Model file for the job. Use its own axes, mm. A direction names the side the tool comes from. Round coordinates to 2 decimals unless told otherwise and drop trailing zeros. Order: outer loops, then holes, each group sorted by start corner. A loop starts at its lowest first (then second) coordinate and runs counter-clockwise, first axis right, second up. Notation, with made-up numbers: M -35,-38.75 L -3,-38.75 A32 ccw -3,-3.75 Z; hole C 62.25,85.5 d3. An arc over 180 degrees is marked long. Return JSON: item names as keys, results as strings. Group by question number.
Item 1: Slice it at C-C on z = 19.05. Write the cut outline in (x, y) (3 decimals).
Item 2: Which spindle directions (+Z, -Z, +X, -X, +Y, -Y) get a long thin tool onto all of the face, cutting with end or side? Do faces 4 (the face through (-3.746, 3.422, -0.165)), 5 (the face through (-0.37, -1.29, 2.85)), 6 (the face through (0, 15.875, 19)). Say none if no direction does.
Item 3: Probe line 1 along Z through (x, y) = (0, 2.15) (3 decimals); line 2 along Z through (x, y) = (0, 3.1) (3 decimals); line 3 along Z through (x, y) = (0, 3.25) (3 decimals). List the from-to ranges inside material, lowest first.
Item 4: Slice it at D-D on y = 13.75. Write the cut outline in (x, z) (3 decimals), then the cut area to 3 significant figures.
Item 5: Pull direction Z, two halves, no side cores. Call faces 1 (the face through (0, 3.175, 7)), 2 (the face through (-4.42, 1.57, 9.59)), 3 (the face through (-1, 3.675, -3)): pulls with the +Z half, pulls with the -Z half, needs draft (parallel to the pull), parting line crosses it, or undercut.
Item 6: Pin check, flat tips, straight feed: pin 1 Ø6 at (x, z) = (-0.5, 1) entering from +Y (3 decimals); pin 2 Ø4.5 at (x, z) = (1, -0.5) entering from -Y; pin 3 Ø5 at (y, z) = (12, 18) entering from +X (3 decimals); pin 4 Ø3 at (y, z) = (5, 3) entering from -X. Stop position of each tip, or through.
Item 7: Slice it at B-B on y = 1. Write the cut outline in (x, z) (3 decimals), then the cut area to 3 significant figures.
Item 8: Slice it at A-A on x = 0. Write the cut outline in (y, z) (3 decimals).
from build123d import *

# Parameters (mm, degrees)
SKETCH1_R           = 1.5
BOSS_EXTRUDE1_DEPTH = 3.175
SKETCH2_R           = 3.75
SKETCH2_R_2         = 2.75
BOSS_EXTRUDE2_DEPTH = 0.5
SKETCH3_R           = 2.75
SKETCH3_R_2         = 1.5
CUT_EXTRUDE1_DEPTH  = 0.8
SKETCH4_R           = 4.5
SKETCH4_R_2         = 2.5
BOSS_EXTRUDE3_DEPTH = 3.048
SKETCH5_R           = 2.875
CUT_EXTRUDE3_DEPTH  = 3.048
SKETCH6_R           = 3.175
BOSS_EXTRUDE4_DEPTH = 12.7
FILLET1_R           = 0.508


with BuildPart() as part:
    # Sketch1 → Boss-Extrude1 (new body)
    with BuildSketch(Plane(origin=(0, 0, 0), x_dir=(1, 0, 0), z_dir=(0, 1, 0))):
        with BuildLine():
            Line((-5.656854249, 0), (-3.148946712, -19.45590591))
            ThreePointArc((-3.148946712, -19.45590591), (0, -22.225), (3.148946712, -19.45590591))
            Line((3.148946712, -19.45590591), (5.656854249, 0))
            ThreePointArc((5.656854249, 0), (0, 5.656854249), (-5.656854249, 0))
        make_face()
        Circle(SKETCH1_R, mode=Mode.SUBTRACT)
    extrude(amount=BOSS_EXTRUDE1_DEPTH)

    # Sketch2 → Boss-Extrude2 (add)
    with BuildSketch(Plane(origin=(0, 3.175, 0), x_dir=(1, 0, 0), z_dir=(0, 1, 0))):
        Circle(SKETCH2_R)
        Circle(SKETCH2_R_2, mode=Mode.SUBTRACT)
    extrude(amount=BOSS_EXTRUDE2_DEPTH)

    # Sketch3 → Cut-Extrude1 (cut)
    with BuildSketch(Plane(origin=(0, 3.675, 0), x_dir=(1, 0, 0), z_dir=(0, 1, 0))):
        Circle(SKETCH3_R)
        Circle(SKETCH3_R_2, mode=Mode.SUBTRACT)
    extrude(amount=-CUT_EXTRUDE1_DEPTH, mode=Mode.SUBTRACT)

    # Sketch4 → Boss-Extrude3 (add)
    with BuildSketch(Plane.XZ):
        Circle(SKETCH4_R)
        Circle(SKETCH4_R_2, mode=Mode.SUBTRACT)
    extrude(amount=BOSS_EXTRUDE3_DEPTH)

    # Sketch5 → Cut-Extrude3 (cut)
    with BuildSketch(Plane.XZ.offset(3.048)):
        Circle(SKETCH5_R)
    extrude(amount=-CUT_EXTRUDE3_DEPTH, mode=Mode.SUBTRACT)

    # Sketch6 → Boss-Extrude4 (add)
    with BuildSketch(Plane(origin=(0, 3.175, 0), x_dir=(1, 0, 0), z_dir=(0, 1, 0))):
        with Locations((0, -19.05)):
            Circle(SKETCH6_R)
    extrude(amount=BOSS_EXTRUDE4_DEPTH)

    # Fillet1
    fillet1_edges = [part.edges().sort_by_distance(p)[0] for p in [
        (-2.875, -3.048, 0),
    ]]
    fillet(fillet1_edges, radius=FILLET1_R)


solid = part.part
Output values:
{
 "1": {"outline": "M -3.201,0 L 3.201,0 L 3.201,3.175 L 3.175,3.175 L 3.175,15.875 L -3.175,15.875 L -3.175,3.175 L -3.201,3.175 Z"},
 "2": {"face 4": "+Y", "face 5": "-Y", "face 6": "+Z, -Z, +X, -X, +Y"},
 "3": {"line 1": "-5.657 to -1.5, 1.5 to 22.225", "line 2": "-5.657 to -2.75, 2.75 to 22.225", "line 3": "-3.75 to -2.75, 2.75 to 3.75, 15.875 to 22.225"},
 "4": {"outline": "C 0,19.05 d6.35", "area": "31.7 mm²"},
 "5": {"face 1": "undercut", "face 2": "pulls with the +Z half", "face 3": "needs draft"},
 "6": {"pin 1": "y = 3.675", "pin 2": "y = -3.05", "pin 3": "x = 3.175", "pin 4": "x = -2.96"},
 "7": {"outline": "M -5.657,0 A5.657 ccw 5.657,0 L 3.149,19.456 A3.175 ccw -3.149,19.456 Z; hole C 0,0 d3", "area": "228 mm²"},
 "8": {"outline": "M -3.048,-4.5 L 0,-4.5 L 0,-5.657 L 3.175,-5.657 L 3.175,-3.75 L 3.675,-3.75 L 3.675,-2.75 L 2.875,-2.75 L 2.875,-1.5 L 0,-1.5 L 0,-2.875 L -2.54,-2.875 A0.508 ccw -3.048,-3.383 Z; M -3.048,3.383 A0.508 ccw -2.54,2.875 L 0,2.875 L 0,1.5 L 2.875,1.5 L 2.875,2.75 L 3.675,2.75 L 3.675,3.75 L 3.175,3.75 L 3.175,15.875 L 15.875,15.875 L 15.875,22.225 L 0,22.225 L 0,4.5 L -3.048,4.5 Z"}
}
